```python
from build123d import *

# Parameters (mm, degrees)
F0_R     = 1.5
F1_DEPTH = 6.25


with BuildPart() as f1:
    # F0 (on Top) → F1 (new body, symmetric)
    with BuildSketch(Plane.XY):
        Circle(F0_R)
    extrude(amount=F1_DEPTH, both=True)

    # F2 (on Front) → F3 (revolve, cut)
    with BuildSketch(Plane.XZ):
        with BuildLine():
            Line((-1.6585878329, 5.95), (-1.5, 5.95))
            ThreePointArc((-1.5, 5.95), (-0.764852927, 6.1742646352), (0, 6.25))
            Line((0, 6.25), (0, 6.3502374105))
            Line((0, 6.3502374105), (-1.6585878329, 6.3502374105))
            Line((-1.6585878329, 6.3502374105), (-1.6585878329, 6.25))
            Line((-1.6585878329, 6.25), (-1.6585878329, 5.95))
        make_face()
    revolve(axis=Axis((0, 0, 3.125), (0, 0, -1)), mode=Mode.SUBTRACT)

    # F4 (on Front) → F5 (revolve, cut)
    with BuildSketch(Plane.XZ):
        Polygon((-0.9272391541, -7.9875725775), (-1.5, -5.85), (-1.5, -7.9875725775), align=None)
    revolve(axis=Axis((0, 0, -6.25), (0, 0, 1)), mode=Mode.SUBTRACT)


solid = f1.part
```
The listing builds one solid part. Answer for the finished solid, in the listing's coordinates (mm). Coordinates: 2 decimals unless noted, no trailing zeros. Write each loop counter-clockwise with the first axis right and the second up, starting at its lowest first coordinate (ties: lowest second). Pieces come first, ordered by that corner, then holes. Notation, with made-up numbers: (32.25, 74) -> (55.25, 74) arc R27 cw to (55.25, 98) -> close; hole circle Ø3 at (0, -7.5). An arc over 180 degrees is marked (long way). Write each question's results on one line, items separated by ' | '. Start each with the question number.
1) A flat-ended cylindrical pin translates along its axis: pin 1 Ø1 at (y, z) = (1, 0.5) entering from +X. Find the tip coordinate at first contact, or state that the pin passes through.
2) A cutting plane is placed at A-A (z = 0.75). Determine the outline of the cut face in (x, y), then the cut area to 3 significant figures.
3) Straight lines are drawn through the part: probe 1 along Y at (x, z) = (-0.1, 5.5); probe 2 along Y at (x, z) = (0.6, 2.5); probe 3 along Z at (x, y) = (-1.3, 0.05). For each, find the intervals that lie inside material, in ascending order.
Values follow:
1) pin 1: x = 1.41
2) outline: circle Ø3 at (0, 0) | area: 7.07 mm²
3) probe 1: -1.5 to 1.5 | probe 2: -1.37 to 1.37 | probe 3: -6.25 to 6.03
